```python
from build123d import *

# Parameters (mm, degrees)
SKETCH1_R               = 25.4
BOSS_EXTRUDE1_DEPTH     = 63.5
FILLET2_R               = 20.32
FILLET3_R               = 12.7
SKETCH2_R               = 13.97
BOSS_EXTRUDE2_DEPTH     = 44.45
SKETCH4_R               = 10.033
CUT_EXTRUDE1_DEPTH      = 50.8
CUT_EXTRUDE2_REACH      = 27.4
CUT_EXTRUDE2_END_RADIUS = 13.97
SKETCH11_R              = 5


with BuildPart() as part:
    # Sketch1 → Boss-Extrude1 (new body)
    with BuildSketch(Plane(origin=(0, 0, 0), x_dir=(1, 0, 0), z_dir=(0, 1, 0))):
        with Locations(Location((0, 0, 0), (0, 0, 270))):  # turned: the seam where the file's is
            Circle(SKETCH1_R)
    extrude(amount=BOSS_EXTRUDE1_DEPTH)

    # Fillet2
    fillet2_edges = [part.edges().sort_by_distance(p)[0] for p in [
        (0, 0, -25.4),
    ]]
    fillet(fillet2_edges, radius=FILLET2_R)

    # Fillet3
    fillet3_edges = [part.edges().sort_by_distance(p)[0] for p in [
        (0, 63.5, -25.4),
    ]]
    fillet(fillet3_edges, radius=FILLET3_R)

    # Sketch2 → Boss-Extrude2 (add)
    with BuildSketch(Plane(origin=(0, 63.5, 0), x_dir=(1, 0, 0), z_dir=(0, 1, 0))):
        with Locations(Location((0, 0, 0), (0, 0, 270))):  # turned: the seam where the file's is
            Circle(SKETCH2_R)
    extrude(amount=BOSS_EXTRUDE2_DEPTH)

    # Sketch4 → Cut-Extrude1 (cut)
    with BuildSketch(Plane(origin=(0, 107.95, 0), x_dir=(1, 0, 0), z_dir=(0, 1, 0))):
        with Locations(Location((0, 0, 0), (0, 0, 270))):  # turned: the seam where the file's is
            Circle(SKETCH4_R)
    extrude(amount=-CUT_EXTRUDE1_DEPTH, mode=Mode.SUBTRACT)

    # Cut-Extrude2: up to this cylinder (the profile starts inside it)
    cut_extrude2_end = Plane(origin=(0, 88.9, 0), z_dir=(0, -1, 0)) * Cylinder(CUT_EXTRUDE2_END_RADIUS, 83.74, mode=Mode.PRIVATE)
    # Sketch11 → Cut-Extrude2 (cut, up to the surface)
    with BuildSketch(Plane.XY, mode=Mode.PRIVATE) as cut_extrude2_sk1:
        with Locations((0, 88.9)):
            Circle(SKETCH11_R)
    cut_extrude2_tool1 = extrude(cut_extrude2_sk1.sketch, amount=-CUT_EXTRUDE2_REACH, mode=Mode.PRIVATE) & cut_extrude2_end
    add(cut_extrude2_tool1.solids().sort_by_distance((0, 88.9, 0))[0], mode=Mode.SUBTRACT)


solid = part.part
```
Input: part model. Units: mm. Frame: model coordinates. A direction names the side the tool comes from. Give positions to 0.01 mm unless a question says otherwise; leave off trailing zeros. Order: outer loops, then holes, each group sorted by start corner. A loop starts at its lowest first (then second) coordinate and runs counter-clockwise, first axis right, second up. Notation, with made-up numbers: (-2, 51) -> (24, 51) arc R30 cw to (24, 80) -> close; hole circle Ø6 at (-15.5, 8). An arc over 180 degrees is marked (long way). Write each question's results on one line, items separated by ' | '. Start each with the question number.
Item 1: Contact query for flat-ended pins moving along their axis: P1, Ø2, axis at x = -6.5, z = 0, coming from the +Y side; P2, Ø8, axis at y = 77.5, z = 19.5, coming from the -X side; P3, Ø5, axis at x = -1.5, z = -9, coming from the +Y side; P4, Ø8, axis at x = 0, y = 88.9, coming from the +Z side. Output: stop coordinate, or through.
Item 2: Line query: line 1 (Z direction, x = 0, y = 75); line 2 (Z direction, x = -1, y = 41); line 3 (X direction, y = 88, z = -10). Output: solid intervals per line, ascending.
Item 3: Set-up query: faces 1 (the cylindrical face through (4.77, 90.4, -11.3)), 2 (the cylindrical face through (-15.456, 35.347, -20.157)). Return all of +Z, -Z, +X, -X, +Y, -Y with unobstructed straight access to the full face (end or side cutting, diameter ignored); none if empty.
Item 4: Cut plane A-A on y = 80. Return the cut outline in (x, z).
Item 5: Mould query, pull axis Z, two halves, no side actions, for faces 3 (the cylindrical face through (3.01, 82.91, 9.57)), 4 (the flat face through (10, 107.95, -3)), 5 (the cylindrical face through (4.196, 85.414, 13.325)), 6 (the flat face through (0, 57.15, 0)). Classes: pulls with the +Z half, pulls with the -Z half, needs draft (parallel to the pull), parting line crosses it, or undercut.
Established:
1) P1: y = 57.15 | P2: through | P3: y = 107.95 | P4: z = 13.97
2) line 1: -13.97 to -10.03, 10.03 to 13.97 | line 2: -25.38 to 25.38 | line 3: -9.76 to -4.92, 4.92 to 9.76
3) face 1: -Z | face 2: +Y, -Y
4) outline: circle Ø27.94 at (0, 0); hole circle Ø20.07 at (0, 0)
5) face 3: undercut | face 4: needs draft | face 5: parting line crosses it | face 6: undercut
